Geometry: final body of the model. Coordinates: model frame, mm. A direction names the side the tool comes from. Give positions to 0.01 mm unless a question says otherwise; leave off trailing zeros. Write each loop counter-clockwise with the first axis right and the second up, starting at its lowest first coordinate (ties: lowest second). Pieces come first, ordered by that corner, then holes. Notation, with made-up numbers: (10, -19) -> (32, -19) arc R21 ccw to (32, 8) -> close; hole circle Ø1 at (69, 39). An arc over 180 degrees is marked (long way). Use CSV: the item, a comma, the result in double quotes. Start each with the question number.
1) Section C-C (z = 6.5). Output: boundary loops of the cut face in (x, y).
2) Contact query for flat-ended pins moving along their axis: P1, Ø1.5, axis at x = 3, z = 9, coming from the -Y side; P2, Ø2, axis at x = 6, z = -1, coming from the +Y side; P3, Ø2, axis at y = 3, z = 13, coming from the +X side. Output: stop coordinate, or through.
3) Material intervals for line 1 (Y direction, x = -5, z = 2) (3 decimals); line 2 (Y direction, x = 0.25, z = 6); line 3 (X direction, y = -7, z = -0.5), sorted ascending. Write a range as [from, to].
4) Draft query along X for faces 1 (the face through (-1.73, -7.81, 9.86)), 2 (the face through (0, 0, 20)), 3 (the face through (-5.158, 3.955, -2.465)). Return one class per face: pulls with the +X half, pulls with the -X half, needs draft (parallel to the pull), parting line crosses it, or undercut.
5) Section A-A (y = 0). Output: boundary loops of the cut face in (x, z), plus the area to 3 significant figures.
6) Set-up query: faces 4 (the face through (-8, -2, 0)), 5 (the face through (0, 0, -5)). Return all of +Z, -Z, +X, -X, +Y, -Y with unobstructed straight access to the full face (end or side cutting, diameter ignored); none if empty.
```python
from build123d import *

# Parameters (mm, degrees)
SKETCH1_R           = 8
BOSS_EXTRUDE1_DEPTH = 20
SKETCH3_R           = 6.5
BOSS_EXTRUDE2_DEPTH = 5


with BuildPart() as part:
    # Sketch1 → Boss-Extrude1 (new body)
    with BuildSketch(Plane.XY):
        Circle(SKETCH1_R)
    extrude(amount=BOSS_EXTRUDE1_DEPTH)

    # Sketch2 → Revolve1 (revolve)
    with BuildSketch(Plane(origin=(0, 0, 0), x_dir=(1, 0, 0), z_dir=(0, 1, 0))):
        with BuildLine():
            Line((9.451478866, 0), (6.548521134, 0))
            ThreePointArc((6.548521134, 0), (8, 1.451478866), (9.451478866, 0))
        make_face()
    revolve(axis=Axis((0, 0, 0), (0, 0, -1)))

    # Sketch3 → Boss-Extrude2 (add)
    with BuildSketch(Plane(origin=(0, 0, 0), x_dir=(-1, 0, 0), z_dir=(0, 0, -1))):
        with Locations(Location((0, 0, 0), (0, 0, 180))):
            Circle(SKETCH3_R)
    extrude(amount=BOSS_EXTRUDE2_DEPTH)


solid = part.part
```
Answers follow:
1,outline,"circle Ø16 at (0, 0)"
2,P1,"stops at y = -7.68"
2,P2,"stops at y = 7.83"
2,P3,"stops at x = 7.75"
3,line 1,"y = [-6.245, 6.245]"
3,line 2,"y = [-8, 8]"
3,line 3,"x = [-6.22, 6.22]"
4,face 1,"parting line crosses it"
4,face 2,"needs draft"
4,face 3,"undercut"
5,outline,"(-9.45, 0) arc R1.45 ccw to (-6.55, 0) -> (-6.5, 0) -> (-6.5, -5) -> (6.5, -5) -> (6.5, 0) -> (6.55, 0) arc R1.45 ccw to (9.45, 0) -> (8, 0) -> (8, 20) -> (-8, 20) -> (-8, 0) -> close"
5,area,"392 mm^2"
6,face 4,"+Z"
6,face 5,"-Z, +X, -X, +Y, -Y"
